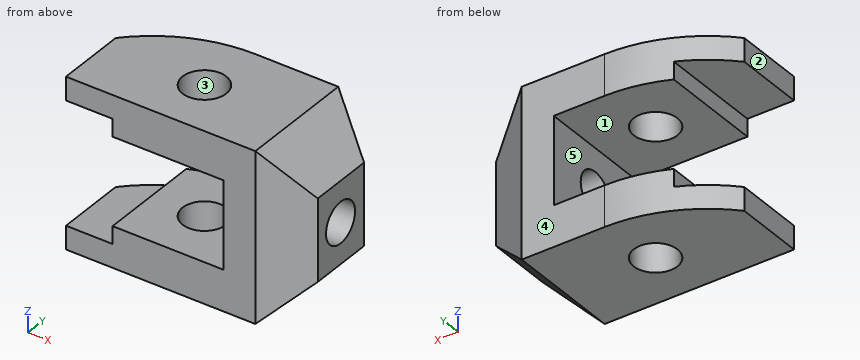
```python
from build123d import *

# Parameters (mm, degrees)
BOSS_EXTRUDE1_DEPTH = 58
SKETCH3_R           = 7.5
CUT_EXTRUDE1_DEPTH  = 107.60206377
CUT_EXTRUDE2_DEPTH  = 107.60206377
CUT_EXTRUDE3_DEPTH  = 107.60206377
SKETCH6_R           = 7
CUT_EXTRUDE4_DEPTH  = 107.60206377


with BuildPart() as part:
    # Sketch2 → Boss-Extrude1 (new body)
    with BuildSketch(Plane.XY):
        with BuildLine():
            Line((0, 0), (65, 0))
            Line((65, 0), (80, 9.029262631))
            Line((80, 9.029262631), (80, 31.339745962))
            Line((80, 31.339745962), (65, 40))
            Line((65, 40), (36.66060556, 40))
            ThreePointArc((36.66060556, 40), (16.66060556, 35.82575695), (0, 24))
            Line((0, 24), (0, 0))
        make_face()
    extrude(amount=-BOSS_EXTRUDE1_DEPTH)

    # Sketch3 → Cut-Extrude1 (cut, through all)
    with BuildSketch(Plane.XY):
        with Locations((34, 19)):
            Circle(SKETCH3_R)
    extrude(amount=-CUT_EXTRUDE1_DEPTH, mode=Mode.SUBTRACT)

    # Sketch4 → Cut-Extrude2 (cut, through all)
    with BuildSketch(Plane(origin=(0, 0, 0), x_dir=(1, 0, 0), z_dir=(0, 1, 0))):
        Polygon((65, 58), (80, 43), (80, 58), align=None)
        Polygon((80, 0), (80, 15), (65, 0), align=None)
    extrude(amount=CUT_EXTRUDE2_DEPTH, mode=Mode.SUBTRACT)

    # Sketch5 → Cut-Extrude3 (cut, through all)
    with BuildSketch(Plane.XZ):
        Polygon((0, -8), (0, -50), (16, -50), (16, -44), (54, -44), (54, -14), (16, -14), (16, -8), align=None)
    extrude(amount=-CUT_EXTRUDE3_DEPTH, mode=Mode.SUBTRACT)

    # Sketch6 → Cut-Extrude4 (cut, through all)
    with BuildSketch(Plane(origin=(80, 0, 0), x_dir=(0, 0, -1), z_dir=(1, 0, 0))):
        with Locations((29, 20)):
            Circle(SKETCH6_R)
    extrude(amount=-CUT_EXTRUDE4_DEPTH, mode=Mode.SUBTRACT)


solid = part.part
```
Source: CAD feature listing. Evaluate the final solid. Frame: model axes, mm. Face numbers are marked on the shaded views. A direction names the side the tool comes from. Give positions to 0.01 mm unless a question says otherwise; leave off trailing zeros. Loops run counter-clockwise (first coordinate to the right, second up) from the corner with the lowest first, then second, coordinate; pieces in that order, holes last. Notation, with made-up numbers: (15, 61.5) -> (32, 61.5) arc R21 cw to (32, 81.5) -> close; hole circle Ø7 at (-6, 80). An arc over 180 degrees is marked (long way). Use a Markdown table: item, result. Add a question column.
(1) Section query A-A (z = -29). Output: boundary loops of the cut face in (x, y).
(2) Access query for the marked faces 4 and 5. Directions: +Z, -Z, +X, -X, +Y, -Y. A direction counts if a zero-diameter tool reaches every point of the face in a straight line with its end or side. Return the directions, or none.
(3) Section query B-B (y = 20). Output: boundary loops of the cut face in (x, z), then the cut area to 3 significant figures.
(4) Section query C-C (x = 11). Output: boundary loops of the cut face in (y, z), then the cut area to 3 significant figures.
(5) Ray query, line 1 (Z direction, x = 7, y = 11); line 2 (Y direction, x = 64.25, z = -29); line 3 (Z direction, x = 34, y = 8.5). Return the intervals inside material, ascending.
(6) Pull-direction query (X, two-part tool) for the marked faces 1, 2 and 3; classes: +X half, -X half, draft (parallel to the pull), parting line (faces both ways), or undercut.
(7) Section query D-D (z = -11). Output: boundary loops of the cut face in (x, y), then the cut area to 3 significant figures.
(8) First-contact query: pin 1 Ø1 at (y, z) = (32, -47.5) entering from -X; pin 2 Ø5 at (x, y) = (71, 32) entering from +Z; pin 3 Ø12.5 at (y, z) = (20, -29) entering from -X; pin 4 Ø1.5 at (y, z) = (14, -50.5) entering from +X. Flat tips, straight axial feed; report the tip coordinate or a pass-through.
Checked values:
| question | item | result |
|---|---|---|
| 1 | outline | (54, 0) -> (65, 0) -> (80, 9.03) -> (80, 13) -> (54, 13) -> close; (54, 27) -> (80, 27) -> (80, 31.34) -> (65, 40) -> (54, 40) -> close |
| 2 | face 4 | +Z, -Z, +X, -X, +Y |
| 2 | face 5 | -X, +Y, -Y |
| 3 | outline | (0, -58) -> (26.57, -58) -> (26.57, -44) -> (16, -44) -> (16, -50) -> (0, -50) -> close; (0, -8) -> (16, -8) -> (16, -14) -> (26.57, -14) -> (26.57, 0) -> (0, 0) -> close; (41.43, -58) -> (65, -58) -> (80, -43) -> (80, -36) -> (54, -36) -> (54, -44) -> (41.43, -44) -> close; (41.43, -14) -> (54, -14) -> (54, -22) -> (80, -22) -> (80, -15) -> (65, 0) -> (41.43, 0) -> close |
| 3 | area | 1,820 mm^2 |
| 4 | outline | (0, -58) -> (32.91, -58) -> (32.91, -50) -> (0, -50) -> close; (0, -8) -> (32.91, -8) -> (32.91, 0) -> (0, 0) -> close |
| 4 | area | 527 mm^2 |
| 5 | line 1 | -58 to -50, -8 to 0 |
| 5 | line 2 | 0 to 13, 27 to 40 |
| 5 | line 3 | -58 to -44, -14 to 0 |
| 6 | face 1 | draft |
| 6 | face 2 | -X half |
| 6 | face 3 | undercut |
| 7 | outline | (16, 0) -> (65, 0) -> (76, 6.62) -> (76, 33.65) -> (65, 40) -> (36.66, 40) arc R50 ccw to (16, 35.53) -> close; hole circle Ø15 at (34, 19) |
| 7 | area | 2,120 mm^2 |
| 8 | pin 1 | x = 16 |
| 8 | pin 2 | z = -3.5 |
| 8 | pin 3 | through |
| 8 | pin 4 | x = 73.25 |
